Could you check a few things on this drawing? It's one solid part, dimensions in mm from its lowest x, y, z. Give positions to 0.01 mm unless a question says otherwise; leave off trailing zeros. Write each loop counter-clockwise with the first axis right and the second up, starting at its lowest first coordinate (ties: lowest second). Pieces come first, ordered by that corner, then holes. Notation, with made-up numbers: (30.25, 54) - (54.25, 54) arc R14 cw to (54.25, 66) - close; hole circle Ø6 at (70.5, -16). An arc over 180 degrees is marked (long way). One line per item, written item: value. Start each with the question number.
1) I'm going to push flat-ended pins straight in: P1, Ø2.5, axis at y = 80.96, z = 12.7, coming from the -X side; P2, Ø1.5, axis at x = 7.5, y = 199, coming from the +Z side (1 decimal). Where does each tip first touch, or does it pass through?
2) We'd pull the mould along X, two halves only. Please class the marked faces 1, 2, 3 and 4: +X half, -X half, draft (parallel to the pull), parting line (faces both ways), or undercut.
3) Please list where these lines run through material, in increasing order: L1, parallel to Y at x = 24.1, z = 12.7 (1 decimal); L2, parallel to X at y = 158, z = 8.5 (1 decimal); L3, parallel to Y at x = 1.5, z = 11.25 (1 decimal). Write a range as [from, to].
4) Imagine slicing it at C-C on x = 19.25. Write out the boundary of the cut face in (y, z) (1 decimal), plus the area to 3 significant figures.
5) Imagine slicing it at B-B on y = 137. Write out the boundary of the cut face in (x, z) (1 decimal).
6) Imagine slicing it at A-A on z = 18.75. Write out the boundary of the cut face in (x, y) (1 decimal), plus the area to 3 significant figures.
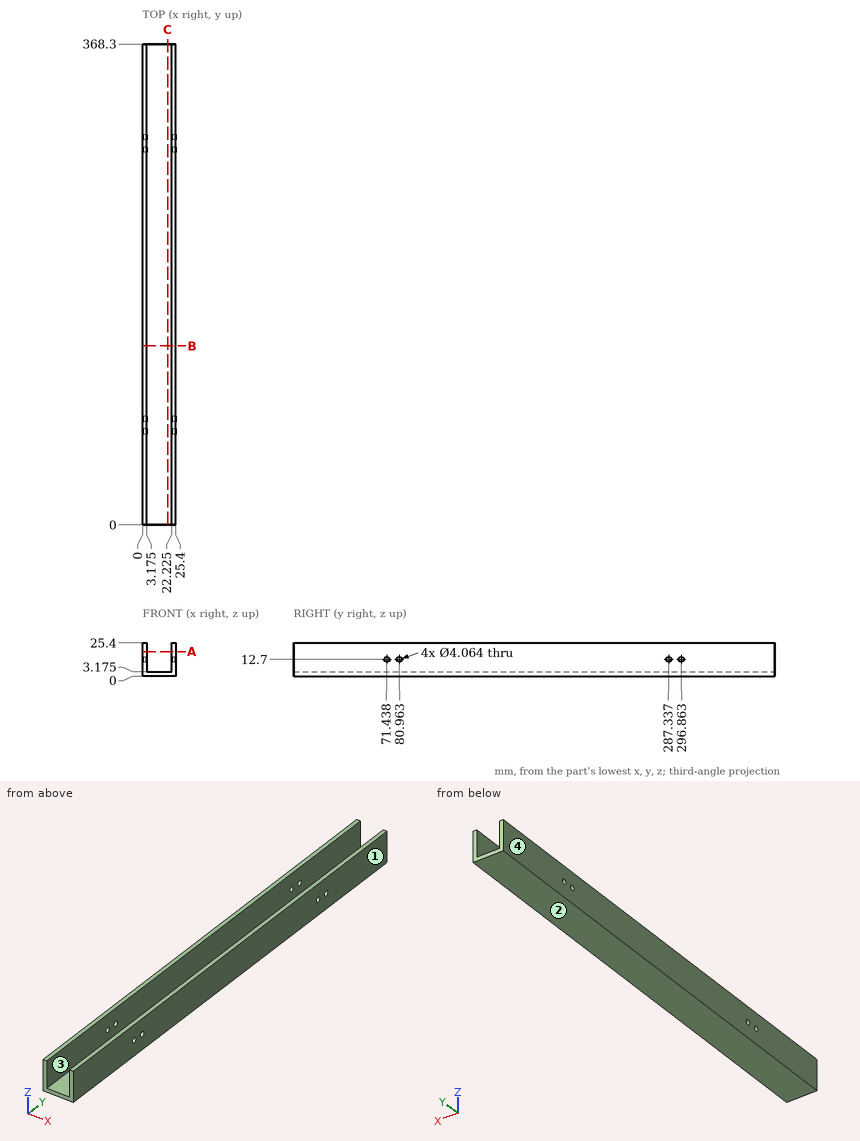
Numbers:
1. P1: through
1. P2: z = 3.2
2. face 1: +X half
2. face 2: draft
2. face 3: undercut
2. face 4: -X half
3. L1: [0, 69.4], [73.5, 78.9], [83, 285.3], [289.4, 294.8], [298.9, 368.3]
3. L2: [0, 3.2], [22.2, 25.4]
3. L3: [0, 70], [72.9, 79.5], [82.4, 285.9], [288.8, 295.4], [298.3, 368.3]
4. outline: (0, 0) - (368.3, 0) - (368.3, 3.2) - (0, 3.2) - close
4. area: 1,170 mm^2
5. outline: (0, 0) - (25.4, 0) - (25.4, 25.4) - (22.2, 25.4) - (22.2, 3.2) - (3.2, 3.2) - (3.2, 25.4) - (0, 25.4) - close
6. outline: (0, 0) - (3.2, 0) - (3.2, 368.3) - (0, 368.3) - close; (22.2, 0) - (25.4, 0) - (25.4, 368.3) - (22.2, 368.3) - close
6. area: 2,340 mm^2
